Autodesk Inventor part; units mm, degrees
ref_plane "YZ Plane" through (0, 0, 0) normal (1, 0, 0) x (0, 1, 0)
ref_plane "XZ Plane" through (0, 0, 0) normal (0, 1, 0) x (-1, 0, 0)
ref_plane "XY Plane" through (0, 0, 0) normal (0, 0, 1) x (1, 0, 0)
sketch "Sketch1" plane through (0, 0, 0) normal (0, 0, 1) x (1, 0, 0)
  circle A0 centre (0, 0) radius 11
  dimension "d0" = 22
extrude "Extrusion1" add sketch "Sketch1" along normal blind 30
sketch "Sketch2" plane through (0, 0, 30) normal (0, 0, 1) x (1, 0, 0)
  circle A0 centre (0, 0) radius 11
  circle A1 centre (0, 0) radius 15
  dimension "d3" = 30
extrude "Extrusion2" add sketch "Sketch2" along normal blind 5 contours A0 | A1
sketch "Sketch6" plane through (0, 0, 35) normal (0, 0, 1) x (1, 0, 0)
  circle A0 centre (0, 0) radius 4
  dimension "d20" = 8
extrude "Extrusion6" add sketch "Sketch6" along normal blind 18
ref_plane "Work Plane1" through (0, 0, 44) normal (0, 0, 1) x (1, 0, 0)
sketch "Sketch7" plane through (0, 0, 44) normal (0, 0, 1) x (1, 0, 0)
  line L0 (1.5, 4) -> (-1.5, 4)
  line L1 (-1.5, 4) -> (-1.5, -4)
  line L2 (-1.5, -4) -> (1.5, -4)
  line L3 (1.5, -4) -> (1.5, 4)
  line L4 (1.5, 4) -> (-1.5, -4) construction
  line L5 (-1.5, 4) -> (1.5, -4) construction
  point P0 (0, 0)
  dimension "d16" = 3
  dimension "d17" = 8
extrude "Extrusion7" cut sketch "Sketch7" along normal blind 3
properties part number "ClickHolder"
Input: part model. Units: mm. Frame: model coordinates. A direction names the side the tool comes from. Coordinates: 2 decimals unless noted, no trailing zeros. Order: outer loops, then holes, each group sorted by start corner. A loop starts at its lowest first (then second) coordinate and runs counter-clockwise, first axis right, second up. Notation, with made-up numbers: M 33,-22.5 L 49,-22.5 A24 ccw 49,-8.5 Z; hole C 34,-36 d1. An arc over 180 degrees is marked long. Answer in a Markdown table with one row per item.
(1) Contact query for flat-ended pins moving along their axis: pin 1 Ø1.5 at (x, y) = (-8, -8.5) entering from +Z; pin 2 Ø8 at (x, z) = (-10.5, 6) entering from +Y; pin 3 Ø3.5 at (y, z) = (1, 46) entering from +X. Output: stop coordinate, or through.
Numbers:
| item | result |
|---|---|
| pin 1 | stops at z = 35 |
| pin 2 | stops at y = 8.87 |
| pin 3 | stops at x = 4 |
(2) Material intervals for line 1 (Z direction, x = -8, y = -9); line 2 (Z direction, x = 5.75, y = 7.25); line 3 (Y direction, x = 3.75, z = 18), sorted ascending. Write a range as [from, to].
Numbers:
| item | result |
|---|---|
| line 1 | z = [30, 35] |
| line 2 | z = [0, 35] |
| line 3 | y = [-10.34, 10.34] |
(3) Draft query along X for faces 6 (the cylindrical face through (-2.38, 10.74, 14.79)), 7 (the flat face through (-1.5, 0, 45)), 8 (the flat face through (0, 0, 47)), 9 (the flat face through (0, 0, 0)). Return one class per face: pulls with the +X half, pulls with the -X half, needs draft (parallel to the pull), parting line crosses it, or undercut.
Numbers:
| item | result |
|---|---|
| face 6 | parting line crosses it |
| face 7 | undercut |
| face 8 | undercut |
| face 9 | needs draft |
(4) Access query for faces 1 (the flat face through (0, 0, 53)), 2 (the cylindrical face through (-14.985, -0.66, 32.465)), 3 (the flat face through (1.5, 0, 45)), 4 (the cylindrical face through (3.695, 1.532, 43.874)), 5 (the flat face through (-5, 10, 30)). Directions: +Z, -Z, +X, -X, +Y, -Y. A direction counts if a zero-diameter tool reaches every point of the face in a straight line with its end or side. Return the directions, or none.
Numbers:
| item | result |
|---|---|
| face 1 | +Z, +X, -X, +Y, -Y |
| face 2 | +Z, -Z |
| face 3 | +Y, -Y |
| face 4 | +Z |
| face 5 | -Z |
(5) Section query B-B, the plane y = 0. Output: boundary loops of the cut face in (x, z), plus the area to 3 significant figures.
Numbers:
| item | result |
|---|---|
| outline | M -15,30 L -11,30 L -11,0 L 11,0 L 11,30 L 15,30 L 15,35 L 4,35 L 4,53 L -4,53 L -4,35 L -15,35 Z; hole M -1.5,44 L 1.5,44 L 1.5,47 L -1.5,47 Z |
| area | 945 mm^2 |
(6) Section query C-C, the plane z = 3. Output: boundary loops of the cut face in (x, y).
Numbers:
| item | result |
|---|---|
| outline | C 0,0 d22 |
(7) Section query D-D, the plane x = -9.75. Output: boundary loops of the cut face in (y, z).
Numbers:
| item | result |
|---|---|
| outline | M -11.4,30 L -5.09,30 L -5.09,0 L 5.09,0 L 5.09,30 L 11.4,30 L 11.4,35 L -11.4,35 Z |
(8) Section query A-A, the plane x = 0. Output: boundary loops of the cut face in (y, z).
Numbers:
| item | result |
|---|---|
| outline | M -15,30 L -11,30 L -11,0 L 11,0 L 11,30 L 15,30 L 15,35 L 4,35 L 4,44 L -4,44 L -4,35 L -15,35 Z; M -4,47 L 4,47 L 4,53 L -4,53 Z |
